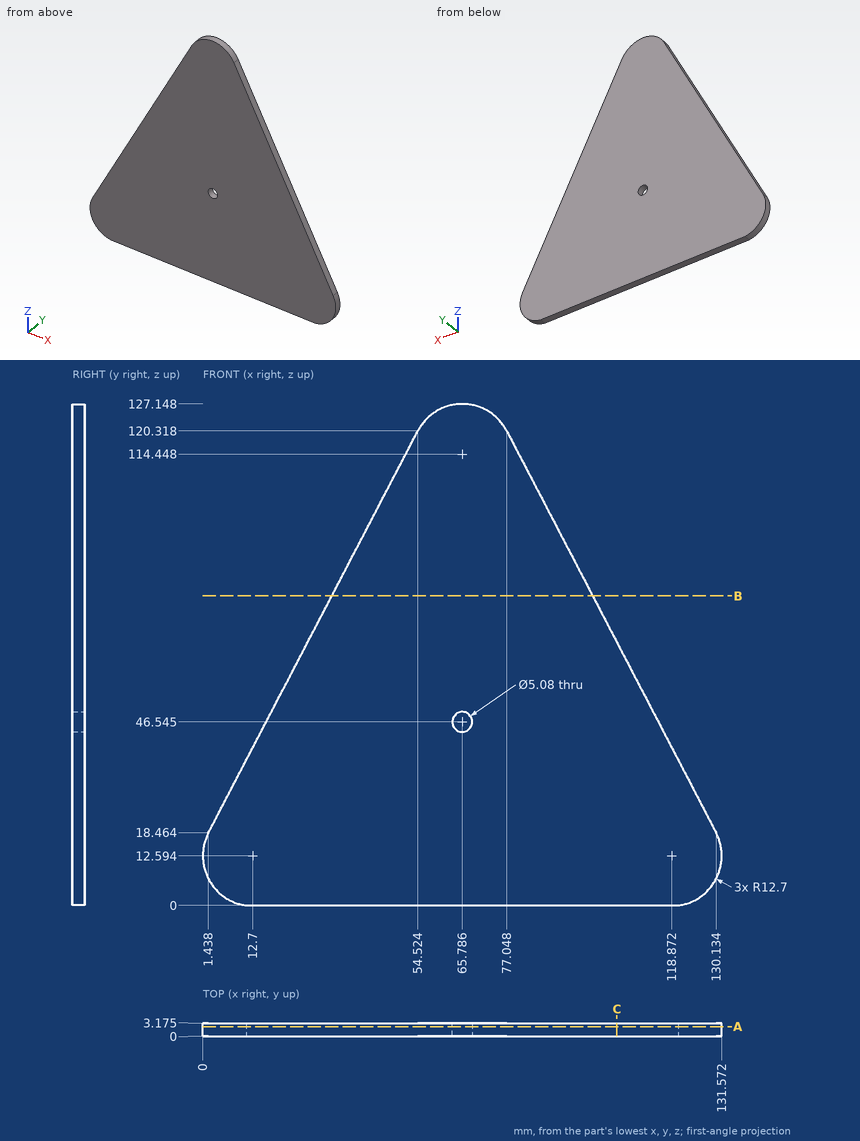
Check sheet for the drawn part. Datum: minimum x, y, z corner. Units: mm. Round coordinates to 2 decimals unless told otherwise and drop trailing zeros. Loops run counter-clockwise (first coordinate to the right, second up) from the corner with the lowest first, then second, coordinate; pieces in that order, holes last. Notation, with made-up numbers: (70, -23.5) - (113, -23.5) arc R27 cw to (113, 10.5) - close; hole circle Ø9 at (-21.5, 60). An arc over 180 degrees is marked (long way). Write each question's results on one line, items separated by ' | '. Start each with the question number.
Q1. Cross-section at B-B on z = 78.5. Enter the section's corners in (x, y) (1 decimal).
Q2. Gauge pin test, flat ends, axial feed: P1, Ø2, axis at x = 49, z = 55.5, coming from the -Y side; P2, Ø12, axis at x = 29, z = 95, coming from the -Y side. Record the tip position at first contact, or that the pin passes through.
Q3. Cross-section at C-C on x = 105. Enter the section's corners in (y, z) (1 decimal), and give its area (3 significant figures).
Q4. Thickness scan on line 1 (Z direction, x = 66, y = 1.7) (1 decimal); line 2 (X direction, y = 2.9, z = 13.5); line 3 (Z direction, x = 57.5, y = 1.1). Record the ranges inside material, lowest first. Write a range as [from, to].
Q5. Cross-section at A-A on y = 2.4. Enter the section's corners in (x, z) (1 decimal), and give its area (3 significant figures).
Answers below:
1) outline: (32.7, 0) - (98.8, 0) - (98.8, 3.2) - (32.7, 3.2) - close
2) P1: stops at y = 0 | P2: passes through
3) outline: (0, 0) - (3.2, 0) - (3.2, 66.7) - (0, 66.7) - close | area: 212 mm²
4) line 1: z = [0, 44], [49.1, 127.1] | line 2: x = [0.03, 131.54] | line 3: z = [0, 124.07]
5) outline: (1.4, 18.5) arc R12.7 ccw to (11.1, 0) - (120.5, 0) arc R12.7 ccw to (130.1, 18.5) - (77, 120.3) arc R12.7 ccw to (54.5, 120.3) - close; hole circle Ø5.1 at (65.8, 46.5) | area: 10,100 mm²
